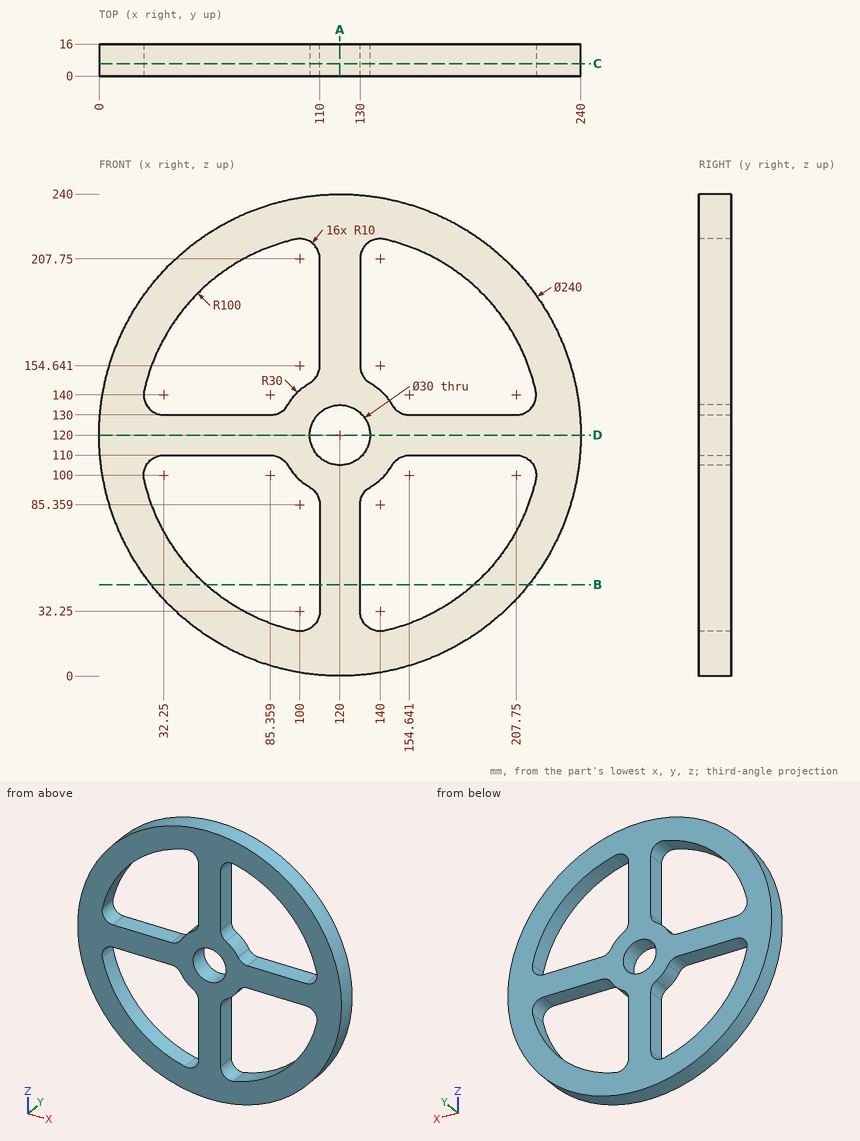
Check sheet for the drawn part. Datum: minimum x, y, z corner. Units: mm. Coordinates: 2 decimals unless noted, no trailing zeros. Order: outer loops, then holes, each group sorted by start corner. A loop starts at its lowest first (then second) coordinate and runs counter-clockwise, first axis right, second up. Notation, with made-up numbers: M 44,-32 L 68,-32 A31 ccw 68,0 Z; hole C 65,55 d4. An arc over 180 degrees is marked long. One line per item, written item: value. Start each with the question number.
Item 1: Gauge pin test, flat ends, axial feed: pin 1 (8 mm diameter, centred on x = 53.5, y = 8.5, fed in from -Z); pin 2 (1.5 mm diameter, centred on y = 4, z = 58, fed in from -X); pin 3 (8 mm diameter, centred on y = 7.5, z = 186, fed in from +X); pin 4 (1.5 mm diameter, centred on x = 213, z = 151, fed in from -Y). Record the tip position at first contact, or that the pin passes through.
Item 2: Sectioned sample at D-D (z = 120). Enter the section's corners in (x, y), then the cut area to 3 significant figures.
Item 3: Sectioned sample at A-A (x = 120). Enter the section's corners in (y, z).
Item 4: Sectioned sample at B-B (z = 45.5). Enter the section's corners in (x, y).
Item 5: Scan lines: probe 1 along Z at (x, y) = (120, 9.5); probe 2 along X at (y, z) = (6.5, 171). Record each from-to range of solid material in increasing order.
Item 6: Sectioned sample at C-C (y = 6.25). Count the separate pieces of the cut face and the enclosed holes in it, then the cut area to 3 significant figures.
Conclusion:
1. pin 1: stops at z = 17.56
1. pin 2: stops at x = 16.81
1. pin 3: stops at x = 222.74
1. pin 4: passes through
2. outline: M 0,0 L 105,0 L 105,16 L 0,16 Z; M 135,0 L 240,0 L 240,16 L 135,16 Z
2. area: 3,360 mm^2
3. outline: M 0,0 L 16,0 L 16,105 L 0,105 Z; M 0,135 L 16,135 L 16,240 L 0,240 Z
4. outline: M 25.93,0 L 53.29,0 L 53.29,16 L 25.93,16 Z; M 110,0 L 130,0 L 130,16 L 110,16 Z; M 186.71,0 L 214.07,0 L 214.07,16 L 186.71,16 Z
5. probe 1: z = 0 to 105, 135 to 240
5. probe 2: x = 11.38 to 33.98, 110 to 130, 206.02 to 228.62
6. separate pieces: 1
6. enclosed holes: 5
6. area: 21,900 mm^2
